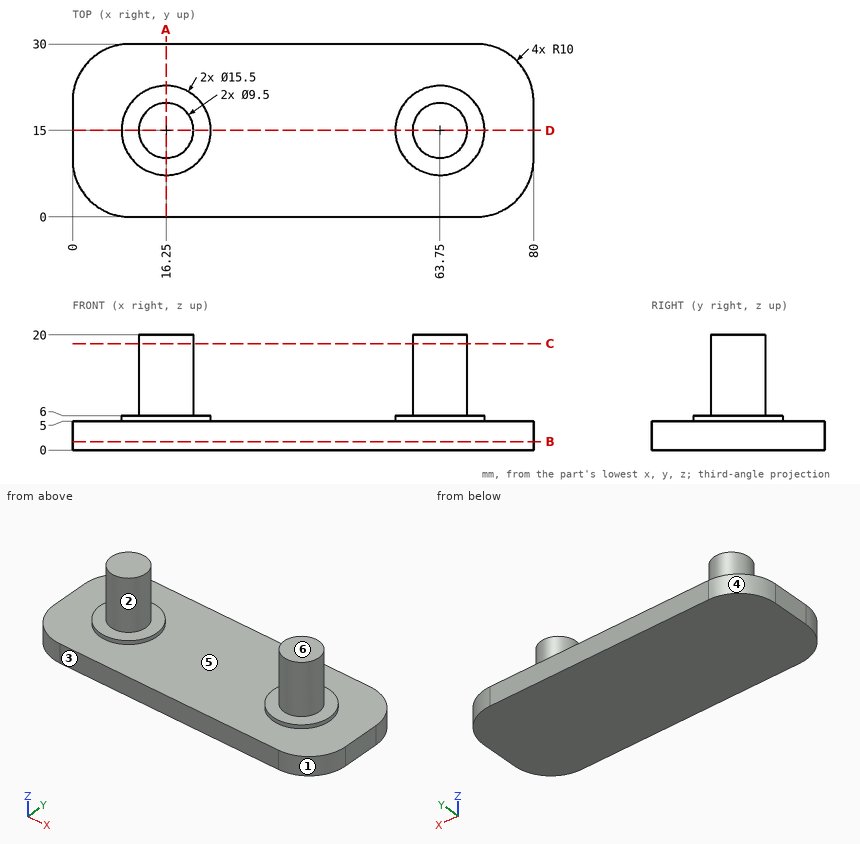
The figure shows three views and two pictorial views of one solid part (mm, origin at its lowest corner). Answer the questions. A direction names the side the tool comes from. Coordinates: 2 decimals unless noted, no trailing zeros. Loops run counter-clockwise (first coordinate to the right, second up) from the corner with the lowest first, then second, coordinate; pieces in that order, holes last.
(1) The mould has two halves that part along X. Classify the marked faces 1, 2, 3 and 4: released by +X, released by -X, zero draft, split by the parting line, or undercut.
Solution:
face 1: released by +X
face 2: undercut
face 3: zero draft
face 4: released by -X
(2) The part is cut by section B-B (z = 1.5). Determine the outline of the cut face in (x, y), and give its area (3 significant figures).
Solution:
outline: (0, 10) arc R10 ccw to (10, 0) - (70, 0) arc R10 ccw to (80, 10) - (80, 20) arc R10 ccw to (70, 30) - (10, 30) arc R10 ccw to (0, 20) - close
area: 2,310 mm2
(3) The part is cut by section D-D (y = 15). Determine the outline of the cut face in (x, z), and give its area (3 significant figures).
Solution:
outline: (0, 0) - (80, 0) - (80, 5) - (71.5, 5) - (71.5, 6) - (68.5, 6) - (68.5, 20) - (59, 20) - (59, 6) - (56, 6) - (56, 5) - (24, 5) - (24, 6) - (21, 6) - (21, 20) - (11.5, 20) - (11.5, 6) - (8.5, 6) - (8.5, 5) - (0, 5) - close
area: 697 mm2
(4) The part is cut by section A-A (x = 16.25). Determine the outline of the cut face in (y, z), and give its area (4 significant figures).
Solution:
outline: (0, 0) - (30, 0) - (30, 5) - (22.75, 5) - (22.75, 6) - (19.75, 6) - (19.75, 20) - (10.25, 20) - (10.25, 6) - (7.25, 6) - (7.25, 5) - (0, 5) - close
area: 298.5 mm2
(5) A tool of negligible diameter and unlimited length cuts with its end or side. For the marked faces 5 and 6, from which of +Z, -Z, +X, -X, +Y, -Y can it reach the whole face along a straight path? Write none if from no direction.
Solution:
face 5: +Z
face 6: +Z, +X, -X, +Y, -Y
(6) Flat-ended cylindrical pins translate along their axes: pin 1 Ø8 at (x, z) = (55.5, 10.5) entering from -Y; pin 2 Ø4 at (y, z) = (17.5, 12.5) entering from -X; pin 3 Ø5 at (y, z) = (8.5, 11) entering from +X. Find the tip coordinate at first contact, or state that the pin passes through.
Solution:
pin 1: stops at y = 12.88
pin 2: stops at x = 11.53
pin 3: stops at x = 66.31
(7) The part is cut by section C-C (z = 18.5). Determine the outline of the cut face in (x, y), and give its area (3 significant figures).
Solution:
outline: circle Ø9.5 at (16.25, 15); circle Ø9.5 at (63.75, 15)
area: 142 mm2
(8) Consider line 1 along Z through (x, y) = (56, 10.5); line 2 along X through (y, z) = (19, 12); line 3 along X through (y, z) = (14, 12.5). Determine where each line is inside the solid, lowest interval first.
Solution:
line 1: z = 0 to 5
line 2: x = 13.69 to 18.81, 61.19 to 66.31
line 3: x = 11.61 to 20.89, 59.11 to 68.39
